Here's how the part is built. I have some questions about the finished solid (model axes, mm). A direction names the side the tool comes from. Coordinates: 2 decimals unless noted, no trailing zeros. Order: outer loops, then holes, each group sorted by start corner. A loop starts at its lowest first (then second) coordinate and runs counter-clockwise, first axis right, second up. Notation, with made-up numbers: (-39.5, 15.25) - (-30.5, 15.25) arc R18 ccw to (-30.5, 41.25) - close; hole circle Ø9 at (-35, 24). An arc over 180 degrees is marked (long way). Answer as CSV lines item,"result". Start each with the question number.
Q1. I need wall thicknesses on line 1 (X direction, y = 58, z = 14); line 2 (X direction, y = -17, z = 47.5); line 3 (Z direction, x = 47, y = 61.5). Which ranges of each line are inside material? Lowest first, please.
Q2. Suppose I cut it at B-B (z = 35). Please give me the cut outline in (x, y), then the cut area to 3 significant figures.
Q3. For faces 1 (the face through (39.5, 60, 67.5)), 2 (the face through (-38.3, -60, 2.5)), 3 (the face through (8.5, -8, 35)), 4 (the face through (-6, 5.9, 67.5)), which set-ups out of +Z, -Z, +X, -X, +Y, -Y let a thin tool reach every point of the face, with its end or its side?
Q4. Suppose I cut it at C-C (y = -65). Please give me the cut outline in (x, z).
Q5. Suppose I cut it at A-A (y = -14.5). Please give me the cut outline in (x, z), then the cut area to 3 significant figures.
Q6. For pin 1 Ø18 at (x, z) = (-29.5, 48.5) entering from +Y; pin 2 Ø18 at (y, z) = (-9, 41.5) entering from +X; pin 3 Ø1.5 at (x, z) = (45.5, 10.5) entering from -Y, each with a flat end and sliding along its axis, tell me the tip position at first contact or that it passes through.
Q7. Suppose I cut it at D-D (z = 60). Please give me the cut outline in (x, y).
Q8. Thinking about a two-plate mould opening in Z: for faces 5 (the face through (74.5, 67.4, 20)), 6 (the face through (5, -74, 3)), 7 (the face through (6, -5.9, 67.5)), 8 (the face through (59.8, 75, 20.5)), which applies, released by +Z, released by -Z, zero draft, split by the parting line, or undercut?
from build123d import *

# Parameters (mm, degrees)
F0_W     = 17
F0_H     = 115
F1_DEPTH = 70
F2_SIZE  = 5
F4_DEPTH = 20.001
F5_SIZE  = 5
F6_SIZE  = 5


with BuildPart() as f1:
    # F0 (on Top) → F1 (new body)
    with BuildSketch(Plane.XY):
        Rectangle(F0_W, F0_H)
        Polygon((-8.5, 57.5), (8.5, 57.5), (76.5, 57.5), (76.5, 77.5), (-8.5, 77.5), align=None)
        Polygon((8.5, -77.5), (8.5, -57.5), (-8.5, -57.5), (-76.5, -57.5), (-76.5, -77.5), align=None)
    extrude(amount=F1_DEPTH)

    # F2
    f2_edges = [f1.edges().sort_by_distance(p)[0] for p in [
        (-8.5, 77.5, 35),
        (-8.5, 10, 70),
        (34, 77.5, 70),
        (-42.5, -57.5, 70),
        (8.5, -10, 70),
        (-34, -77.5, 70),
        (42.5, 57.5, 70),
        (34, 77.5, 0),
        (42.5, 57.5, 0),
        (8.5, -10, 0),
        (-34, -77.5, 0),
        (8.5, -77.5, 35),
        (-42.5, -57.5, 0),
        (-8.5, 10, 0),
    ]]
    chamfer(f2_edges, length=F2_SIZE)

    # F3 (on face) → F4 (cut, through all)
    with BuildSketch(Plane.XZ.offset(-57.5)):
        with BuildLine():
            Line((43.5, 23), (43.5, 47))
            ThreePointArc((43.5, 47), (31.5, 35), (43.5, 23))
        make_face()
        with BuildLine():
            ThreePointArc((43.5, 23), (51.9852813742, 26.5147186258), (55.5, 35))
            ThreePointArc((55.5, 35), (51.9852813742, 43.4852813742), (43.5, 47))
            Line((43.5, 47), (43.5, 23))
        make_face()
        with BuildLine():
            ThreePointArc((43.5, 47), (51.9852813742, 43.4852813742), (55.5, 35))
            ThreePointArc((55.5, 35), (51.9852813742, 26.5147186258), (43.5, 23))
            Line((43.5, 23), (76.5, 23))
            Line((76.5, 23), (76.5, 47))
            Line((76.5, 47), (43.5, 47))
        make_face()
    extrude(amount=-F4_DEPTH, mode=Mode.SUBTRACT)

    # F5
    f5_edges = [f1.edges().sort_by_distance(p)[0] for p in [
        (31.5, 57.5, 35),
        (31.5, 77.5, 35),
        (76.5, 67.5, 47),
        (76.5, 67.5, 23),
    ]]
    chamfer(f5_edges, length=F5_SIZE)

    # F6 (call 1 of 6: OpenCascade refuses the feature's edges together)
    f6_edges = [f1.edges().sort_by_distance(p)[0] for p in [
        (76.5, 67.5, 70),
    ]]
    chamfer(f6_edges, length=F6_SIZE)

    # F6#2 (call 2 of 6)
    f6_2_edges = [f1.edges().sort_by_distance(p)[0] for p in [
        (76.5, 67.5, 0),
    ]]
    chamfer(f6_2_edges, length=F6_SIZE)

    # F6#3 (call 3 of 6)
    f6_3_edges = [f1.edges().sort_by_distance(p)[0] for p in [
        (-76.5, -57.5, 35),
    ]]
    chamfer(f6_3_edges, length=F6_SIZE)

    # F6#4 (call 4 of 6)
    f6_4_edges = [f1.edges().sort_by_distance(p)[0] for p in [
        (-76.5, -77.5, 35),
    ]]
    chamfer(f6_4_edges, length=F6_SIZE)

    # F6#5 (call 5 of 6)
    f6_5_edges = [f1.edges().sort_by_distance(p)[0] for p in [
        (-76.5, -67.5, 0),
    ]]
    chamfer(f6_5_edges, length=F6_SIZE)

    # F6#6 (call 6 of 6)
    f6_6_edges = [f1.edges().sort_by_distance(p)[0] for p in [
        (-76.5, -67.5, 70),
    ]]
    chamfer(f6_6_edges, length=F6_SIZE)


solid = f1.part
Here are the results:
1,line 1,"x = -8.5 to 76.5"
1,line 2,"x = -8.5 to 8.5"
1,line 3,"z = 1 to 22, 48 to 69"
2,outline,"(-76.5, -72.5) - (-71.5, -77.5) - (3.5, -77.5) - (8.5, -72.5) - (8.5, 57.5) - (26.5, 57.5) - (31.5, 62.5) - (31.5, 72.5) - (26.5, 77.5) - (-3.5, 77.5) - (-8.5, 72.5) - (-8.5, -57.5) - (-71.5, -57.5) - (-76.5, -62.5) - close"
2,area,"4,380 mm²"
3,face 1,"+Z, +X, -Y"
3,face 2,"-Z, -X, +Y"
3,face 3,"+Z, -Z, +X, -Y"
3,face 4,"+Z, -X, +Y"
4,outline,"(-76.5, 5) - (-71.5, 0) - (3.5, 0) - (8.5, 5) - (8.5, 65) - (3.5, 70) - (-71.5, 70) - (-76.5, 65) - close"
5,outline,"(-8.5, 5) - (-3.5, 0) - (3.5, 0) - (8.5, 5) - (8.5, 65) - (3.5, 70) - (-3.5, 70) - (-8.5, 65) - close"
5,area,"1,140 mm²"
6,pin 1,"stops at y = -57.5"
6,pin 2,"stops at x = 8.5"
6,pin 3,"stops at y = 57.5"
7,outline,"(-76.5, -72.5) - (-71.5, -77.5) - (3.5, -77.5) - (8.5, -72.5) - (8.5, 57.5) - (76.5, 57.5) - (76.5, 77.5) - (-3.5, 77.5) - (-8.5, 72.5) - (-8.5, -57.5) - (-71.5, -57.5) - (-76.5, -62.5) - close"
8,face 5,"undercut"
8,face 6,"released by -Z"
8,face 7,"released by +Z"
8,face 8,"undercut"
